For this review, take the finished solid that the model builds, in its own axes (mm). Round coordinates to 2 decimals unless told otherwise and drop trailing zeros. Write each loop counter-clockwise with the first axis right and the second up, starting at its lowest first coordinate (ties: lowest second). Pieces come first, ordered by that corner, then holes. Notation, with made-up numbers: (-14.5, 35) -> (-0.5, 35) arc R6 ccw to (-0.5, 46) -> close; hole circle Ø2 at (28.5, 59.25). An arc over 180 degrees is marked (long way). Answer in a Markdown table with one row per item. Add a question column.
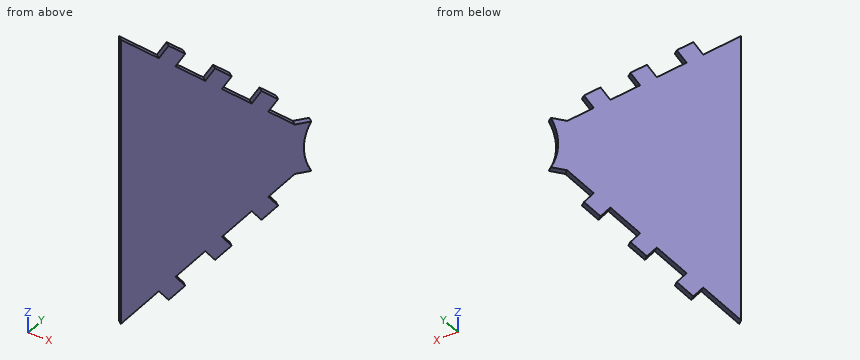
Autodesk Inventor part; units mm, degrees
ref_plane "Work Plane1" through (-64.6593, -63.2457, 0) normal (-0.788, 0.6157, 0) x (-0.6157, -0.788, 0)
ref_plane "YZ Plane" through (0, 0, 0) normal (1, 0, 0) x (0, 1, 0)
ref_plane "XZ Plane" through (0, 0, 0) normal (0, 1, 0) x (-1, 0, 0)
sketch "Sketch1" plane through (0, 0, 0) normal (0, 0, 1) x (1, 0, 0)
  line L0 (-27.3641, -15.51) -> (-92.3641, -98.7062)
  line L1 (-26.8641, -15.51) -> (-26.8641, 15.51)
  line L2 (-26.8641, -15.51) -> (-27.3641, -15.51) construction
  line L3 (-54.6593, -71.0586) -> (-64.6593, -63.2457)
  point P0 (0, 0)
  dimension "d0" = 0.5
  dimension "d1" = 38
  dimension "d2" = 65
  dimension "d3" = 10
  dimension "d4" = 45
ref_plane "Work Plane1" through (-64.6593, -63.2457, 0) normal (-0.788, 0.6157, 0) x (-0.6157, -0.788, 0)
sketch "Sketch3" plane through (-64.6593, -63.2457, 0) normal (-0.788, 0.6157, 0) x (-0.6157, -0.788, 0)
  line L0 (25.703, 78.6272) -> (-56.7377, 13.663)
  line L1 (-60.5775, 15.51) -> (-60.5775, 13.663) construction
  line L2 (-56.7377, 13.663) -> (-60.5775, 13.663)
  line L3 (-60.5775, 13.663) -> (-60.5775, 0)
  line L4 (25.703, 78.6272) -> (-56.7377, 13.663)
  line L5 (-56.7377, 13.663) -> (-60.5775, 15.51) construction
  line L6 (-60.5775, 15.51) -> (25.703, 83.5) construction
  line L7 (25.703, 78.6272) -> (25.703, 0)
  line L8 (-89.6466, 0) -> (36.1638, 0) construction
  line L9 (25.703, 83.5) -> (25.703, 78.6272) construction
  line L10 (25.703, -78.6272) -> (-56.7377, -13.663)
  line L11 (-56.7377, -13.663) -> (-60.5775, -13.663)
  line L12 (-60.5775, -13.663) -> (-60.5775, 0)
  line L13 (25.703, -78.6272) -> (25.703, 0)
  point P0 (0, 0)
extrude "Extrusion1" add sketch "Sketch3" along normal blind 3
sketch "Sketch4" plane through (-64.6593, -63.2457, 0) normal (0.788, -0.6157, 0) x (0, 0, -1)
  line L0 (-78.6272, -25.703) -> (-13.663, 56.7377)
  line L1 (-23.566, 44.1706) -> (-29.4568, 48.8126)
  line L2 (-29.4568, 48.8126) -> (-35.6462, 40.9582)
  line L3 (-35.6462, 40.9582) -> (-29.7554, 36.3162)
  line L4 (-13.663, 60.5775) -> (13.663, 60.5775) construction
  line L5 (-78.6272, -25.703) -> (-13.663, 56.7377) construction
  line L6 (-52.9764, 18.9659) -> (-47.0856, 14.3238)
  line L7 (-46.787, 26.8203) -> (-52.9764, 18.9659)
  line L8 (-40.8962, 22.1783) -> (-46.787, 26.8203)
  line L9 (-70.3066, -3.0265) -> (-64.4158, -7.6685)
  line L10 (-64.1172, 4.8279) -> (-70.3066, -3.0265)
  line L11 (-58.2264, 0.1859) -> (-64.1172, 4.8279)
  point P0 (0, 89.6466)
  point P1 (-47.0856, 14.3238)
  point P2 (-40.8962, 22.1783)
  dimension "d10" = 7.5
  dimension "d11" = 10
  dimension "d13" = 16
  dimension "d16" = 28
extrude "Extrusion2" add sketch "Sketch4" against normal up to surface (3 mm away)
mirror "Mirror1" about plane through (0, 0, 0) normal (0, 0, 1) of "Extrusion2"
sketch "Sketch6" plane through (-64.6593, -63.2457, 0) normal (0.788, -0.6157, 0) x (0, 0, -1)
  arc A0 (4.4093, 61.3896) -> (-4.4093, 61.3896) centre (0, 89.6466) ccw
  ellipse E0 centre (0, 80.26) end of major axis (0, 60.5775) minor radius 15.51 (4.4093, 61.3896) -> (11.5479, 67.1205) ccw construction
  arc A1 (11.5479, 67.1205) -> (-11.5479, 67.1205) centre (0, 89.6466) ccw construction
  ellipse E1 centre (0, 80.26) end of major axis (0, 60.5775) minor radius 15.51 (-11.5479, 67.1205) -> (-4.4093, 61.3896) ccw construction
  line L0 (-13.663, 56.7377) -> (-13.663, 60.5775)
  line L1 (-13.663, 60.5775) -> (-13.663, 64.5225)
  line L2 (13.663, 60.5775) -> (13.663, 56.7377)
  line L3 (13.663, 60.5775) -> (13.663, 64.5225)
  circle A2 centre (0, 89.6466) radius 28.5989
  line L4 (-13.663, 60.5775) -> (13.663, 60.5775)
  point P0 (0, 89.6466)
  point P1 (4.4093, 61.3896)
  point P2 (-4.4093, 61.3896)
extrude "Extrusion3" add sketch "Sketch6" against normal up to surface (3 mm away) contours A0 L3 L4 L1 A2
properties part number "Tolva_Corto"
1. We need section B-B (z = -0.5). Write out the cut boundary in (x, y), plus the area to 3 significant figures.
2. For L1, parallel to Y at x = -79.5, z = -27; L2, parallel to Y at x = -65, z = -7; L3, parallel to Z at x = -29, y = -17, list the stretches that pass through material, from the lowest coordinate up. Write a range as [from, to].
3. Clearance check with flat-ended pins moving along their axes: pin 1 Ø6 at (x, z) = (-40.5, 29) entering from +Y; pin 2 Ø3 at (x, z) = (-67.5, 29.5) entering from +Y; pin 3 Ø6 at (x, z) = (-52, -30) entering from +Y. State where each tip first meets the part, or that it passes through.
4. We need section A-A (z = -51). Write out the cut boundary in (x, y), plus the area to 3 significant figures.
Response:
| question | item | result |
|---|---|---|
| 1 | outline | (-82.85, -81.65) -> (-80.48, -83.5) -> (-27.07, -15.14) -> (-29.44, -13.29) -> close |
| 1 | area | 260 mm2 |
| 2 | L1 | [-82.24, -77.37] |
| 2 | L2 | [-63.68, -58.81] |
| 2 | L3 | [-13.66, 13.66] |
| 3 | pin 1 | y = -23.61 |
| 3 | pin 2 | y = -60.09 |
| 3 | pin 3 | y = -38.33 |
| 4 | outline | (-82.85, -81.65) -> (-80.48, -83.5) -> (-58.9, -55.87) -> (-61.26, -54.03) -> close; (-56.31, -47.68) -> (-53.94, -49.53) -> (-51.44, -46.32) -> (-53.8, -44.48) -> close |
| 4 | area | 117 mm2 |
